Could you check a few things on this model? Use its own coordinates, in mm. Face numbers are marked on the shaded views. A direction names the side the tool comes from. Give positions to 0.01 mm unless a question says otherwise; leave off trailing zeros. Loops run counter-clockwise (first coordinate to the right, second up) from the corner with the lowest first, then second, coordinate; pieces in that order, holes last. Notation, with made-up numbers: (7, 20) -> (56, 20) arc R17 ccw to (56, 53) -> close; hole circle Ø4 at (-25.5, 54.5). An arc over 180 degrees is marked (long way). Write each question's results on one line, items separated by ' | '. Start each with the question number.
Q1. If I drill on line 1 along Z through (x, y) = (-65, 2.5); line 2 along X through (y, z) = (2.25, 80); line 3 along Y through (x, z) = (91, 38), over which ranges is the centre line in solid material (lowest first)?
Q2. If we section it at A-A, the plane x = 60.5: List the corners of the cut face in (y, z) for me, plus the area to 3 significant figures.
Q3. Will these pins go through, and if not, where does the flat tip stop? P1, Ø3.5, axis at x = -80, z = 65, coming from the +Y side; P2, Ø10, axis at x = -11.5, y = 18, coming from the +Z side; P3, Ø4, axis at x = 24, y = 21.5, coming from the -Z side; P4, Ø1.5, axis at x = 43.5, y = 13, coming from the -Z side.
Q4. We'd pull the mould along Z, two halves only. Please class the marked faces 1 and 2: released by +Z, released by -Z, zero draft, split by the parting line, or undercut.
Q5. Which directions (+Z, -Z, +X, -X, +Y, -Y) give clear straight access to the entire face, cutting with the end or side of a thin tool? Please do the marked faces 3 and 4.
Q6. If we section it at B-B, the plane z = 41: List the corners of the cut face in (x, y) for me.
from build123d import *

# Parameters (mm, degrees)
PLATE_DEPTH         = 9
SKETCH2_R           = 1.09
CASTER_HOLES_DEPTH  = 128.597021909
SKETCH3_R           = 1.6
HEX_HOLES_DEPTH     = 128.597021909
SKETCH4_W           = 20
SKETCH4_H           = 5
BOSS_EXTRUDE1_DEPTH = 20
SKETCH5_W           = 56.7
SKETCH5_H           = 14
BOSS_EXTRUDE2_DEPTH = 3
SKETCH6_R           = 10
CUT_EXTRUDE1_DEPTH  = 24.8
CUT_EXTRUDE2_START  = -24.8
SKETCH7_R           = 10
CUT_EXTRUDE2_DEPTH  = 24.8
SKETCH8_R           = 6
BOSS_EXTRUDE4_DEPTH = 3


with BuildPart() as part:
    # Sketch1 → Plate (new body)
    with BuildSketch(Plane(origin=(0, 0, 0), x_dir=(1, 0, 0), z_dir=(0, 1, 0))):
        with BuildLine():
            Line((-65, -90), (65, -90))
            ThreePointArc((65, -90), (82.67766953, -82.67766953), (90, -65))
            Line((90, -65), (90, 65))
            ThreePointArc((90, 65), (82.67766953, 82.67766953), (65, 90))
            Line((65, 90), (-65, 90))
            ThreePointArc((-65, 90), (-82.67766953, 82.67766953), (-90, 65))
            Line((-90, 65), (-90, -65))
            ThreePointArc((-90, -65), (-82.67766953, -82.67766953), (-65, -90))
        make_face()
    extrude(amount=PLATE_DEPTH)

    # Sketch2 → Caster Holes (cut, through all)
    with BuildSketch(Plane(origin=(0, 9, 0), x_dir=(1, 0, 0), z_dir=(0, 1, 0))):
        with Locations(Location((-7.747, 70, 0), (0, 0, 270))):
            Circle(SKETCH2_R)
        with Locations(Location((7.747, 70, 0), (0, 0, 270))):
            Circle(SKETCH2_R)
    extrude(amount=-CASTER_HOLES_DEPTH, mode=Mode.SUBTRACT)

    # Sketch3 → Hex Holes (cut, through all)
    with BuildSketch(Plane(origin=(0, 9, 0), x_dir=(1, 0, 0), z_dir=(0, 1, 0))):
        with Locations(Location((-65, 80, 0), (0, 0, 270))):
            Circle(SKETCH3_R)
        with Locations(Location((-80, 65, 0), (0, 0, 270))):
            Circle(SKETCH3_R)
        with Locations(Location((80, 65, 0), (0, 0, 270))):
            Circle(SKETCH3_R)
        with Locations(Location((80, -65, 0), (0, 0, 270))):
            Circle(SKETCH3_R)
        with Locations(Location((65, 80, 0), (0, 0, 270))):
            Circle(SKETCH3_R)
        with Locations(Location((65, -80, 0), (0, 0, 270))):
            Circle(SKETCH3_R)
        with Locations(Location((-65, -80, 0), (0, 0, 270))):
            Circle(SKETCH3_R)
        with Locations(Location((-80, -65, 0), (0, 0, 270))):
            Circle(SKETCH3_R)
    extrude(amount=-HEX_HOLES_DEPTH, mode=Mode.SUBTRACT)

    # Sketch4 → Boss-Extrude1 (add)
    with BuildSketch(Plane(origin=(0, 9, 0), x_dir=(1, 0, 0), z_dir=(0, 1, 0))):
        Polygon((-27, -90), (-27, -80), (-22, -80), (-22, -85), (-17, -85), (-17, -90), align=None)
        Polygon((17, -90), (17, -85), (22, -85), (22, -80), (27, -80), (27, -90), align=None)
        with Locations((0, 56)):
            Rectangle(SKETCH4_W, SKETCH4_H)
    extrude(amount=BOSS_EXTRUDE1_DEPTH)

    # Sketch5 → Boss-Extrude2 (add)
    with BuildSketch(Plane(origin=(0, 9, 0), x_dir=(1, 0, 0), z_dir=(0, 1, 0))):
        with Locations((-61.65, -38)):
            Rectangle(SKETCH5_W, SKETCH5_H)
        with Locations((61.65, -38)):
            Rectangle(SKETCH5_W, SKETCH5_H)
    extrude(amount=BOSS_EXTRUDE2_DEPTH)

    # Sketch6 → Cut-Extrude1 (cut)
    with BuildSketch(Plane.ZY.offset(90)):
        with Locations((38, 19.5)):
            Circle(SKETCH6_R)
    extrude(amount=-CUT_EXTRUDE1_DEPTH, mode=Mode.SUBTRACT)

    # Sketch7 → Cut-Extrude2 (cut)
    with BuildSketch(Plane(origin=(90, 0, 0), x_dir=(0, 0, -1), z_dir=(1, 0, 0)).offset(CUT_EXTRUDE2_START)):
        with Locations((-38, 19.5)):
            Circle(SKETCH7_R)
    extrude(amount=CUT_EXTRUDE2_DEPTH, mode=Mode.SUBTRACT)

    # Sketch8 → Boss-Extrude4 (add)
    with BuildSketch(Plane(origin=(90, 0, 0), x_dir=(0, 0, -1), z_dir=(1, 0, 0))):
        with BuildLine():
            Line((-48, 19.5), (-48, 0))
            Line((-48, 0), (-28, 0))
            Line((-28, 0), (-28, 19.5))
            ThreePointArc((-28, 19.5), (-38, 29.5), (-48, 19.5))
        make_face()
        with Locations((-38, 19.5)):
            Circle(SKETCH8_R, mode=Mode.SUBTRACT)
    extrude(amount=BOSS_EXTRUDE4_DEPTH)


solid = part.part
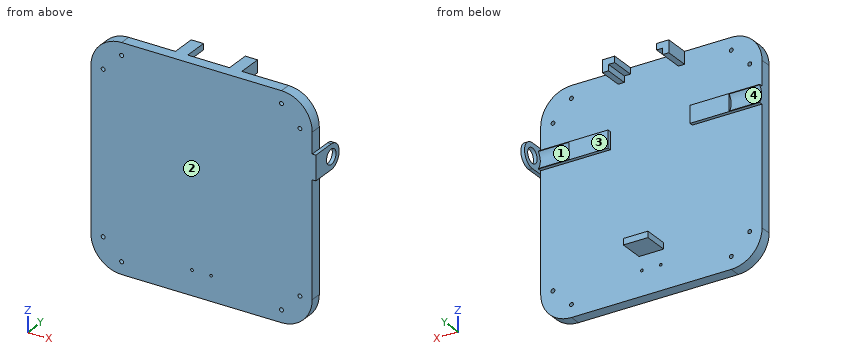
Final values:
1) line 1: z = -90 to -81.6, -78.4 to 78.4, 81.6 to 90 | line 2: x = -85 to -66.6, -63.4 to 63.4, 66.6 to 85 | line 3: y = 0 to 13.5, 25.5 to 29.5
2) outline: (0, -90) -> (9, -90) -> (9, 31) -> (12, 31) -> (12, 45) -> (9, 45) -> (9, 90) -> (0, 90) -> close | area: 1,660 mm²
3) P1: stops at y = 9 | P2: stops at z = -53.5 | P3: stops at z = 80 | P4: passes through
4) face 1: undercut | face 2: zero draft
5) face 3: +Z, -Z, -X, +Y | face 4: -X, +Y
6) outline: (-90, 0) -> (93, 0) -> (93, 14.3) -> (90, 14.3) -> (90, 9.96) -> (65.2, 9.96) -> (65.2, 12) -> (33.3, 12) -> (33.3, 9) -> (-33.3, 9) -> (-33.3, 12) -> (-65.2, 12) -> (-65.2, 9.96) -> (-90, 9.96) -> close; (90, 24.7) -> (93, 24.7) -> (93, 29.04) -> (90, 29.04) -> close
